The listing builds one solid part. Answer for the finished solid, in the listing's coordinates (mm). Face numbers are marked on the shaded views. Give positions to 0.01 mm unless a question says otherwise; leave off trailing zeros. Order: outer loops, then holes, each group sorted by start corner. A loop starts at its lowest first (then second) coordinate and runs counter-clockwise, first axis right, second up. Notation, with made-up numbers: (12.5, -24.5) - (70.5, -24.5) arc R10 cw to (70.5, -14.5) - close; hole circle Ø9 at (34.5, 20.5). An arc over 180 degrees is marked (long way). Answer as CSV lines item,"result". Start each with the question number.
1. Consider line 1 along Z through (x, y) = (8.5, -2.25); line 2 along X through (y, z) = (-6.5, 0.25); line 3 along Z through (x, y) = (-2, -9). Determine where each line is inside the solid, lowest interval first. Write a range as [from, to].
2. Flat-ended cylindrical pins translate along their axes: pin 1 (1 mm diameter, centred on x = -33.5, z = 1, fed in from -Y); pin 2 (8 mm diameter, centred on x = -9.5, z = -4, fed in from +Y); pin 3 (6 mm diameter, centred on y = -1, z = -4, fed in from +X). Find the tip coordinate at first contact, or state that the pin passes through.
3. Section A-A on x = -18 is taken. Give the vertices of the cut face in (y, z), and give its area (3 significant figures).
4. Determine the mould class of the marked faces 1, 2 and 3 for opening direction X: +X half, -X half, draft (parallel to the pull), parting line (faces both ways), or undercut.
5. Section B-B on x = -2 is taken. Give the vertices of the cut face in (y, z), and give its area (3 significant figures).
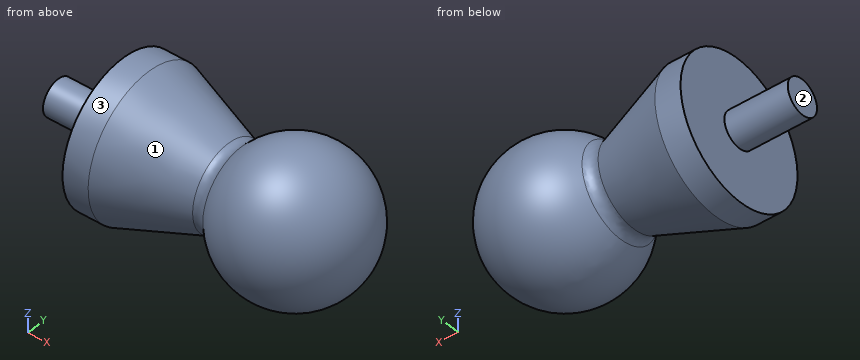
from build123d import *

# Parameters (mm, degrees)
FILLET1_R = 2


with BuildPart() as part:
    # Sketch1 → Revolve1 (revolve)
    with BuildSketch(Plane(origin=(0, 0, 0), x_dir=(1, 0, 0), z_dir=(0, 1, 0))):
        with BuildLine():
            Line((-25, 12), (-10.017761944, 6.6063943))
            ThreePointArc((-10.017761944, 6.6063943), (3.448685016, 11.493762294), (12, 0))
            Line((12, 0), (-40, 0))
            Line((-40, 0), (-40, 3))
            Line((-40, 3), (-29.32, 3))
            Line((-29.32, 3), (-29.32, 12))
            Line((-29.32, 12), (-25, 12))
        make_face()
    revolve(axis=Axis((25.002810952, 0, 0), (-1, 0, 0)))

    # Fillet1
    fillet1_edges = [part.edges().sort_by_distance(p)[0] for p in [
        (-10.017761944, 0, 6.6063943),
    ]]
    fillet(fillet1_edges, radius=FILLET1_R)


solid = part.part
Checks:
1,line 1,"z = [-8.17, 8.17]"
1,line 2,"x = [-29.32, 10.08]"
1,line 3,"z = [-7.68, 7.68]"
2,pin 1,"stops at y = -2.96"
2,pin 2,"stops at y = 10.21"
2,pin 3,"stops at x = 11.95"
3,outline,"circle Ø18.96 at (0, 0)"
3,area,"282 mm²"
4,face 1,"undercut"
4,face 2,"-X half"
4,face 3,"draft"
5,outline,"circle Ø23.66 at (0, 0)"
5,area,"440 mm²"
